The model under review builds one solid part; all positions refer to its coordinate system, in mm. Face numbers are marked on the shaded views. A direction names the side the tool comes from. Coordinates: 2 decimals unless noted, no trailing zeros. Write each loop counter-clockwise with the first axis right and the second up, starting at its lowest first coordinate (ties: lowest second). Pieces come first, ordered by that corner, then holes. Notation, with made-up numbers: (-31, 70.25) - (-2, 70.25) arc R12 ccw to (-2, 87.25) - close; hole circle Ø8 at (1.5, -25.5). An arc over 180 degrees is marked (long way). Return JSON: item names as keys, results as strings. Group by question number.
(1) Draft analysis for pull direction X (two halves, no side actions). For the marked faces 1, 2, 3 and 4, state which applies: released by +X, released by -X, zero draft, split by the parting line, or undercut.
(2) We need section A-A on z = 12.25. State the section outline as (x, y) points (3 decimals), then the cut area to 3 significant figures.
(3) For pin 1 Ø5 at (y, z) = (-5.5, 12.5) entering from -X (3 decimals); pin 2 Ø0.9 at (y, z) = (1.5, 4.5) entering from +X; pin 3 Ø4 at (x, z) = (32, -12.25) entering from -Y; pin 4 Ø3 at (x, z) = (-32, 12.25) entering from -Y, all flat-tipped, find the tip position at first contact; note any pin that passes through.
(4) To check wall thickness, follow L1, parallel to X at y = 0.7, z = 12.25; L2, parallel to Y at x = 6, z = -7.5; L3, parallel to X at y = -5.25, z = 13.5 (3 decimals). State the ranges of each line that lie inside material, in increasing order. Write a range as from..to.
(5) We need section B-B on x = 31. State the section outline as (y, z) points.
(6) Tool access review of the marked faces 5, 6 and 7: name each direction out of +Z, -Z, +X, -X, +Y, -Y from which nothing blocks a thin tool from reaching the whole face with its end or side.
(7) We need section C-C on y = -9. State the section outline as (x, z) points (3 decimals), then the cut area to 3 significant figures.
(8) We need section D-D on x = 5. State the section outline as (y, z) points (3 decimals), then the cut area to 3 significant figures.
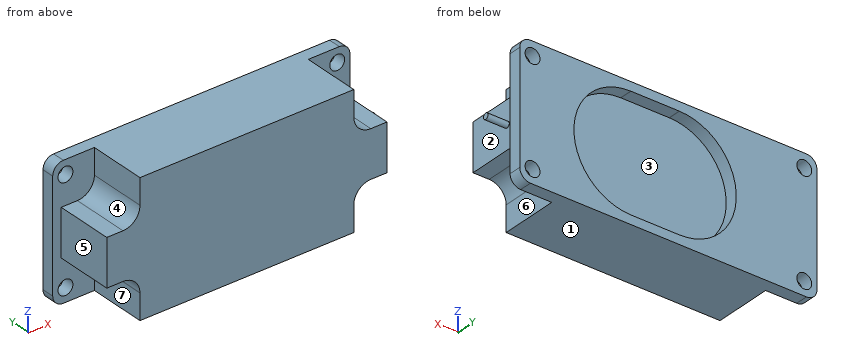
```python
from build123d import *

# Parameters (mm, degrees)
SKETCH1_W           = 70
SKETCH1_H           = 31
SKETCH1_R           = 1.75
BOSS_EXTRUDE1_DEPTH = 2.9
FILLET1_R           = 2.5
BOSS_EXTRUDE2_DEPTH = 13.6
FILLET2_R           = 4
CUT_EXTRUDE1_DEPTH  = 3
SKETCH4_R           = 0.691032606
BOSS_EXTRUDE3_DEPTH = 5


with BuildPart() as part:
    # Sketch1 → Boss-Extrude1 (new body)
    with BuildSketch(Plane(origin=(0, 0, 0), x_dir=(1, 0, 0), z_dir=(0, 1, 0))):
        Rectangle(SKETCH1_W, SKETCH1_H)
        with Locations(Location((-32, 12.25, 0), (0, 0, 270))):
            Circle(SKETCH1_R, mode=Mode.SUBTRACT)
        with Locations(Location((-32, -12.25, 0), (0, 0, 270))):
            Circle(SKETCH1_R, mode=Mode.SUBTRACT)
        with Locations(Location((32, -12.25, 0), (0, 0, 270))):
            Circle(SKETCH1_R, mode=Mode.SUBTRACT)
        with Locations(Location((32, 12.25, 0), (0, 0, 270))):
            Circle(SKETCH1_R, mode=Mode.SUBTRACT)
    extrude(amount=BOSS_EXTRUDE1_DEPTH)

    # Fillet1
    fillet1_edges = [part.edges().sort_by_distance(p)[0] for p in [
        (-35, 1.45, -15.5),
        (35, 1.45, -15.5),
        (35, 1.45, 15.5),
        (-35, 1.45, 15.5),
    ]]
    fillet(fillet1_edges, radius=FILLET1_R)

    # Sketch2 → Boss-Extrude2 (add)
    with BuildSketch(Plane.XZ):
        Polygon((-25.185, -15.5), (25.185, -15.5), (25.185, -5.5), (33, -5.5), (33, 5.5), (25.185, 5.5), (25.185, 15.5), (-25.185, 15.5), (-25.185, 5.5), (-33, 5.5), (-33, -5.5), (-25.185, -5.5), align=None)
    extrude(amount=BOSS_EXTRUDE2_DEPTH)

    # Fillet2
    fillet2_edges = [part.edges().sort_by_distance(p)[0] for p in [
        (25.185, -6.8, 5.5),
        (-25.185, -6.8, 5.5),
        (-25.185, -6.8, -5.5),
        (25.185, -6.8, -5.5),
    ]]
    fillet(fillet2_edges, radius=FILLET2_R)

    # Sketch3 → Cut-Extrude1 (cut)
    with BuildSketch(Plane(origin=(0, 2.9, 0), x_dir=(1, 0, 0), z_dir=(0, 1, 0))):
        with BuildLine():
            Line((-2.575, 13.415), (8.835, 13.415))
            ThreePointArc((8.835, 13.415), (22.25, 0), (8.835, -13.415))
            Line((8.835, -13.415), (-2.575, -13.415))
            ThreePointArc((-2.575, -13.415), (-15.99, 0), (-2.575, 13.415))
        make_face()
    extrude(amount=-CUT_EXTRUDE1_DEPTH, mode=Mode.SUBTRACT)

    # Sketch4 → Boss-Extrude3 (add)
    with BuildSketch(Plane(origin=(33, 0, 0), x_dir=(0, 0, -1), z_dir=(1, 0, 0))):
        with Locations(Location((0, -3.46433499, 0), (0, 0, 180))):
            Circle(SKETCH4_R)
    extrude(amount=BOSS_EXTRUDE3_DEPTH)


solid = part.part
```
Ans:
{
 "1": {"face 1": "zero draft", "face 2": "released by +X", "face 3": "undercut", "face 4": "released by -X"},
 "2": {"outline": "(-35, 0) - (-33.75, 0) - (-33.75, 2.9) - (-35, 2.9) - close; (-30.25, 0) - (-25.185, 0) - (-25.185, -13.6) - (25.185, -13.6) - (25.185, 0) - (30.25, 0) - (30.25, 2.9) - (14.303, 2.9) - (14.303, -0.1) - (-8.043, -0.1) - (-8.043, 2.9) - (-30.25, 2.9) - close; (33.75, 0) - (35, 0) - (35, 2.9) - (33.75, 2.9) - close", "area": "801 mm²"},
 "3": {"pin 1": "x = -25.185", "pin 2": "x = 35", "pin 3": "y = 0", "pin 4": "through"},
 "4": {"L1": "-35..-33.75, -30.25..-8.04, 14.3..30.25, 33.75..35", "L2": "-13.6..-0.1", "L3": "-25.185..25.185"},
 "5": {"outline": "(-13.6, -5.5) - (0, -5.5) - (0, -10.81) - (2.9, -10.81) - (2.9, 10.81) - (0, 10.81) - (0, 5.5) - (-13.6, 5.5) - close; (0, -15.5) - (2.9, -15.5) - (2.9, -13.69) - (0, -13.69) - close; (0, 13.69) - (2.9, 13.69) - (2.9, 15.5) - (0, 15.5) - close"},
 "6": {"face 5": "+Z, -Z, -X, -Y", "face 6": "-Z, +X, -Y", "face 7": "-Z, -X, -Y"},
 "7": {"outline": "(-33, -5.5) - (-29.185, -5.5) arc R4 cw to (-25.185, -9.5) - (-25.185, -15.5) - (25.185, -15.5) - (25.185, -9.5) arc R4 cw to (29.185, -5.5) - (33, -5.5) - (33, 5.5) - (29.185, 5.5) arc R4 cw to (25.185, 9.5) - (25.185, 15.5) - (-25.185, 15.5) - (-25.185, 9.5) arc R4 cw to (-29.185, 5.5) - (-33, 5.5) - close", "area": "1,750 mm²"},
 "8": {"outline": "(-13.6, -15.5) - (2.9, -15.5) - (2.9, -13.415) - (-0.1, -13.415) - (-0.1, 13.415) - (2.9, 13.415) - (2.9, 15.5) - (-13.6, 15.5) - close", "area": "431 mm²"}
}
